Can you work these out from the model? Positions are in its coordinate system, mm. A direction names the side the tool comes from. Give positions to 0.01 mm unless a question says otherwise; leave off trailing zeros. Order: outer loops, then holes, each group sorted by start corner. A loop starts at its lowest first (then second) coordinate and runs counter-clockwise, first axis right, second up. Notation, with made-up numbers: M 5.5,29 L 36.5,29 A16 cw 36.5,43 Z; hole C 33.25,60.5 d3. An arc over 180 degrees is marked long. Use a Markdown table: item, result. Add a question column.
from build123d import *

# Parameters (mm, degrees)
F0_W     = 5
F0_H     = 5
F1_DEPTH = 6
F2_R     = 1.25
F3_DEPTH = 2.5


with BuildPart() as f1:
    # F0 (on Top) → F1 (new body, symmetric)
    with BuildSketch(Plane.XY):
        Rectangle(F0_W, F0_H)
    extrude(amount=F1_DEPTH, both=True)

    # F2 (on face) → F3 (join)
    with BuildSketch(Plane.XY.offset(6)):
        Circle(F2_R)
    extrude(amount=F3_DEPTH)

    # F4: F1 across plane


with BuildPart() as f1_1:
    add(f1.part)
    add(f1.part.mirror(Plane.XY))


solid = f1_1.part
1. If we section it at A-A, the plane y = 0: List the corners of the cut face in (x, z) for me.
2. I need wall thicknesses on L1, parallel to Z at x = 1.3, y = 0.35; L2, parallel to X at y = -1, z = 6.5; L3, parallel to Y at x = 0.7, z = 7. Which ranges of each line are inside material? Lowest first, please. Write a range as [from, to].
3. On a 3-axis mill with a long thin cutter (end or side, diameter ignored), from which of +Z, -Z, +X, -X, +Y, -Y can I reach the whole of each face in a straight line? I mean faces 1 (the face through (0, -2.5, 0)), 2 (the face through (-1, 1, -6)), 3 (the face through (-0.27, -1.22, 7.23)). Say none if no direction works.
4. If we section it at C-C, the plane z = 6.5: List the corners of the cut face in (x, y) for me, then the cut area to 3 significant figures.
5. Will this pin go through, and if not, where does the flat tip stop? pin 1 (1 mm diameter, centred on x = -2, y = 0, fed in from +Z).
Geometry results:
| question | item | result |
|---|---|---|
| 1 | outline | M -2.5,-6 L -1.25,-6 L -1.25,-8.5 L 1.25,-8.5 L 1.25,-6 L 2.5,-6 L 2.5,6 L 1.25,6 L 1.25,8.5 L -1.25,8.5 L -1.25,6 L -2.5,6 Z |
| 2 | L1 | z = [-6, 6] |
| 2 | L2 | x = [-0.75, 0.75] |
| 2 | L3 | y = [-1.04, 1.04] |
| 3 | face 1 | +Z, -Z, +X, -X, -Y |
| 3 | face 2 | -Z |
| 3 | face 3 | +Z |
| 4 | outline | C 0,0 d2.5 |
| 4 | area | 4.91 mm^2 |
| 5 | pin 1 | stops at z = 6 |
